Could you check a few things on this model? Use its own coordinates, in mm. Give positions to 0.01 mm unless a question says otherwise; leave off trailing zeros. Loops run counter-clockwise (first coordinate to the right, second up) from the corner with the lowest first, then second, coordinate; pieces in that order, holes last.
1. Thinking about a two-plate mould opening in Y: for faces 1 (the cylindrical face through (13.39, 39.88, 5.15)), 2 (the flat face through (13, 56.595, 26)), 3 (the flat face through (13, 17, 0)), 4 (the flat face through (13, -21.519, 26)), which applies, +Y half, -Y half, draft (parallel to the pull), parting line (faces both ways), or undercut?
2. Imagine slicing it at A-A (y = -3). List the corners of the cut face in (x, z) for me, plus the area to 3 significant figures.
3. I need wall thicknesses on line 1 along Y through (x, z) = (12.5, 9); line 2 along Z through (x, y) = (23, 42.5); line 3 along X through (y, z) = (25, 5.5). Which ranges of each line are inside material? Lowest first, please.
```python
from build123d import *

# Parameters (mm, degrees)
F0_W     = 78.1140327454
F0_H     = 52.0444214344
F1_DEPTH = 25.4
F2_R     = 7.62
F3_R     = 7.62
F5_D     = 6.35
F5_DEPTH = 10.16
F5_TIP   = 1.9077324654


with BuildPart() as f1:
    # F0 (on Right) → F1 (new body)
    with BuildSketch(Plane.YZ):
        with Locations((17.5377391279, 26.0222107172)):
            Rectangle(F0_W, F0_H)
    extrude(amount=F1_DEPTH)

    # F2
    f2_edges = [f1.edges().sort_by_distance(p)[0] for p in [
        (0, 17.537739, 0),
    ]]
    fillet(f2_edges, radius=F2_R)

    # F3
    f3_edges = [f1.edges().sort_by_distance(p)[0] for p in [
        (25.4, 17.537739, 0),
    ]]
    fillet(f3_edges, radius=F3_R)

    # F5
    with Locations(Plane(origin=(0, 0, 0), x_dir=(1, 0, 0), z_dir=(0, 0, -1))):
        with Locations((12.7, -36.7818512022)):
            Hole(F5_D / 2, depth=F5_DEPTH)
            with Locations((0, 0, -(F5_DEPTH + F5_TIP / 2))):  # 118° drill point
                Cone(0, F5_D / 2, F5_TIP, mode=Mode.SUBTRACT)


solid = f1.part
```
Derived:
1. face 1: undercut
1. face 2: +Y half
1. face 3: draft
1. face 4: -Y half
2. outline: (0, 7.62) arc R7.62 ccw to (7.62, 0) - (17.78, 0) arc R7.62 ccw to (25.4, 7.62) - (25.4, 52.04) - (0, 52.04) - close
2. area: 1,300 mm2
3. line 1: y = -21.52 to 33.61, 39.95 to 56.59
3. line 2: z = 2.07 to 52.04
3. line 3: x = 0.3 to 25.1
